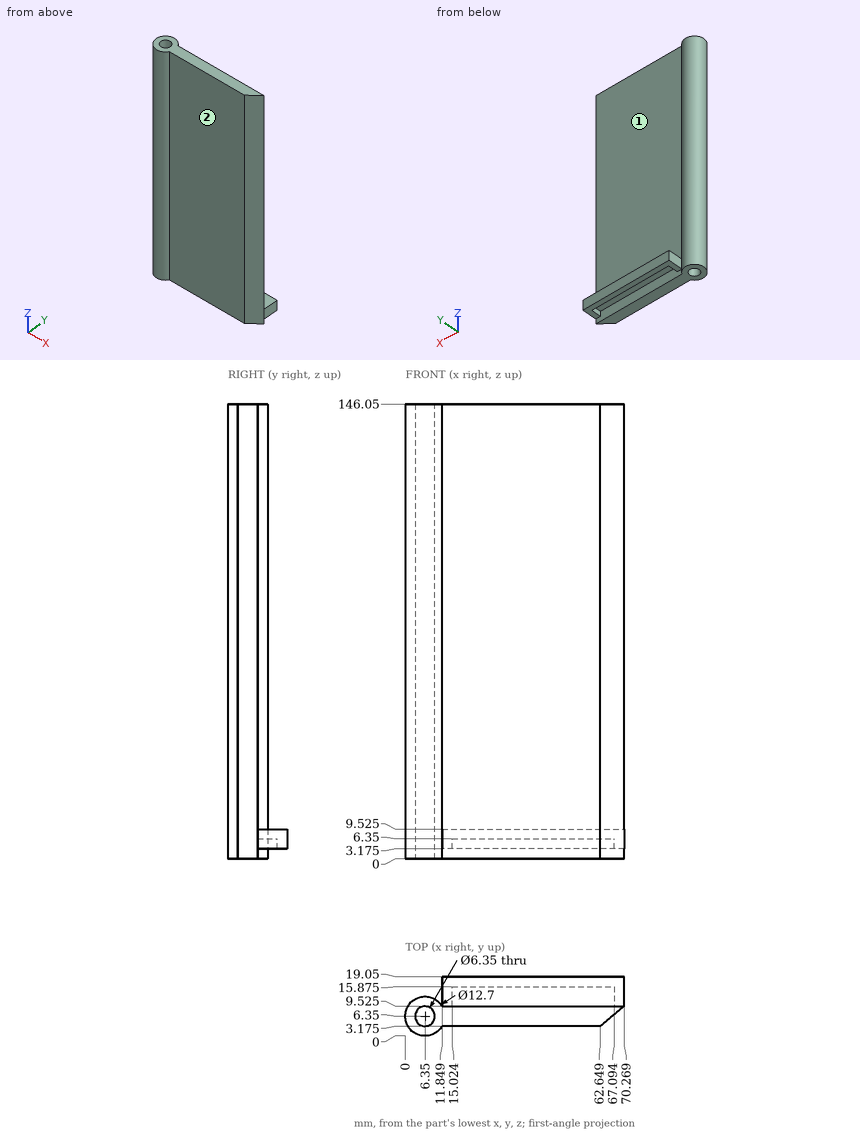
Verification items for this drawing (mm, ordinates from the low corner). A direction names the side the tool comes from. Give positions to 0.01 mm unless a question says otherwise; leave off trailing zeros. Answer as a JSON object with one key per item and string values. Group by question number.
Item 1: Material ranges on L1, parallel to Y at x = 6, z = 110 (1 decimal); L2, parallel to Z at x = 38, y = 16.25 (1 decimal); L3, parallel to X at y = 7.5, z = 66.5 (1 decimal), recorded low to high.
Item 2: Gauge pin test, flat ends, axial feed: pin 1 (4 mm diameter, centred on x = 42, y = 17, fed in from +Z) (3 decimals); pin 2 (17.5 mm diameter, centred on x = 41.5, z = 94.5, fed in from +Y) (3 decimals); pin 3 (5 mm diameter, centred on x = 35, y = 14, fed in from -Z) (3 decimals); pin 4 (6 mm diameter, centred on y = 16.5, z = 91, fed in from -X). Record the tip position at first contact, or that the pin passes through.
Item 3: Access from +Z, -Z, +X, -X, +Y, -Y to the whole of each face (thin tool, end or side, straight path). Record for the marked faces 1 and 2.
Findings below:
{
 "1": {"L1": "0 to 3.2, 9.5 to 12.7", "L2": "3.2 to 9.5", "L3": "0.1 to 3.4, 9.3 to 67.8"},
 "2": {"pin 1": "z = 9.525", "pin 2": "y = 9.525", "pin 3": "z = 3.175", "pin 4": "through"},
 "3": {"face 1": "+Z, +X, +Y", "face 2": "+Z, -Z, +X, -Y"}
}
